from build123d import *

# Parameters (mm, degrees)
SKETCH1_W           = 50
SKETCH1_H           = 50
BOSS_EXTRUDE1_DEPTH = 1439.7
SKETCH2_W           = 50
SKETCH2_H           = 60
BOSS_EXTRUDE2_DEPTH = 100
SKETCH3_W           = 250
SKETCH3_H           = 60
SKETCH3_W_2         = 50
BOSS_EXTRUDE3_DEPTH = 15
SKETCH4_R           = 10
CUT_EXTRUDE1_DEPTH  = 1474.001542864
SKETCH5_R           = 15
CUT_EXTRUDE2_DEPTH  = 1477.156207783
SKETCH7_R           = 15
CUT_EXTRUDE3_DEPTH  = 1477.156207783


with BuildPart() as part:
    # Sketch1 → Boss-Extrude1 (new body)
    with BuildSketch(Plane(origin=(0, 0, 0), x_dir=(1, 0, 0), z_dir=(0, 1, 0))):
        with Locations((-56.349206349, -14.484126984)):
            Rectangle(SKETCH1_W, SKETCH1_H)
    extrude(amount=BOSS_EXTRUDE1_DEPTH)

    # Sketch2 → Boss-Extrude2 (add)
    with BuildSketch(Plane(origin=(-31.349206349, 0, 0), x_dir=(0, 0, -1), z_dir=(1, 0, 0))):
        with Locations((-14.484126984, 1409.7)):
            Rectangle(SKETCH2_W, SKETCH2_H)
        with Locations((-14.484126984, 30)):
            Rectangle(SKETCH2_W, SKETCH2_H)
    extrude(amount=BOSS_EXTRUDE2_DEPTH)

    # Sketch3 → Boss-Extrude3 (add)
    with BuildSketch(Plane(origin=(68.650793651, 0, 0), x_dir=(0, 0, -1), z_dir=(1, 0, 0))):
        with Locations((-164.484126984, 30)):
            Rectangle(SKETCH3_W, SKETCH3_H)
        with Locations((135.515873016, 30)):
            Rectangle(SKETCH3_W, SKETCH3_H)
        with Locations((-164.484126984, 1409.7)):
            Rectangle(SKETCH3_W, SKETCH3_H)
        with Locations((135.515873016, 1409.7)):
            Rectangle(SKETCH3_W, SKETCH3_H)
        with Locations((-14.484126984, 1409.7)):
            Rectangle(SKETCH3_W_2, SKETCH3_H)
        with Locations((-14.484126984, 30)):
            Rectangle(SKETCH3_W_2, SKETCH3_H)
    extrude(amount=BOSS_EXTRUDE3_DEPTH)

    # Sketch4 → Cut-Extrude1 (cut, through all)
    with BuildSketch(Plane.XY.offset(39.484126984)):
        with Locations((-56.577927761, 597.467393714)):
            Circle(SKETCH4_R)
        with Locations((-56.577927761, 527.467393714)):
            Circle(SKETCH4_R)
        with Locations((-56.577927761, 457.467393714)):
            Circle(SKETCH4_R)
        with Locations((-56.577927761, 387.467393714)):
            Circle(SKETCH4_R)
        with Locations((-56.577927761, 317.467393714)):
            Circle(SKETCH4_R)
        with Locations((-56.577927761, 247.467393714)):
            Circle(SKETCH4_R)
        with Locations((-56.577927761, 177.467393714)):
            Circle(SKETCH4_R)
        with Locations((-56.577927761, 107.467393714)):
            Circle(SKETCH4_R)
        with Locations((-56.577927761, 667.467393714)):
            Circle(SKETCH4_R)
        with Locations((-56.577927761, 737.467393714)):
            Circle(SKETCH4_R)
    extrude(amount=-CUT_EXTRUDE1_DEPTH, mode=Mode.SUBTRACT)

    # Sketch5 → Cut-Extrude2 (cut, through all)
    with BuildSketch(Plane.ZY.offset(-68.650793651)):
        with Locations((-228.539538752, 1409.7)):
            Circle(SKETCH5_R)
        with Locations((-168.539538752, 1409.7)):
            Circle(SKETCH5_R)
        with Locations((-108.539538752, 1409.7)):
            Circle(SKETCH5_R)
        with Locations((-48.539538752, 1409.7)):
            Circle(SKETCH5_R)
        with Locations((247.647169752, 1409.7)):
            Circle(SKETCH5_R)
        with Locations((187.647169752, 1409.7)):
            Circle(SKETCH5_R)
        with Locations((127.647169752, 1409.7)):
            Circle(SKETCH5_R)
        with Locations((67.647169752, 1409.7)):
            Circle(SKETCH5_R)
    extrude(amount=-CUT_EXTRUDE2_DEPTH, mode=Mode.SUBTRACT)

    # Sketch7 → Cut-Extrude3 (cut, through all)
    with BuildSketch(Plane.ZY.offset(-68.650793651)):
        with Locations((-230.917241816, 30)):
            Circle(SKETCH7_R)
        with Locations((-170.917241816, 30)):
            Circle(SKETCH7_R)
        with Locations((-110.917241816, 30)):
            Circle(SKETCH7_R)
        with Locations((-50.917241816, 30)):
            Circle(SKETCH7_R)
        with Locations(Location((78.601472043, 30, 0), (0, 0, 180))):
            Circle(SKETCH7_R)
        with Locations(Location((138.601472043, 30, 0), (0, 0, 180))):
            Circle(SKETCH7_R)
        with Locations(Location((198.601472043, 30, 0), (0, 0, 180))):
            Circle(SKETCH7_R)
        with BuildLine():
            ThreePointArc((259.111313866, 44.991332873), (244.62115569, 30), (259.111313866, 15.008667127))
            ThreePointArc((259.111313866, 15.008667127), (273.601472043, 30), (259.111313866, 44.991332873))
        make_face()
    extrude(amount=-CUT_EXTRUDE3_DEPTH, mode=Mode.SUBTRACT)


solid = part.part
The model under review builds one solid part; all positions refer to its coordinate system, in mm. A direction names the side the tool comes from. Round coordinates to 2 decimals unless told otherwise and drop trailing zeros. Write each loop counter-clockwise with the first axis right and the second up, starting at its lowest first coordinate (ties: lowest second). Pieces come first, ordered by that corner, then holes. Notation, with made-up numbers: M 22.25,52 L 49.25,52 A13 cw 49.25,61 Z; hole C 60,-13.75 d10. An arc over 180 degrees is marked long. Answer as CSV lines item,"result". Start each with the question number.
Q1. Wall thickness on line 1 along Y through (x, z) = (26.5, -2); line 2 along Z through (x, y) = (-67, 657.5); line 3 along X through (y, z) = (94, -3): over which ranges is each line inside the solid? List them lowest first.
Q2. Tool access review of faces 1 (the face through (-40, 716, 39.484)), 2 (the face through (51, 1379.7, 16)), 3 (the face through (68.651, 1410, -134)): name each direction out of +Z, -Z, +X, -X, +Y, -Y from which nothing blocks a thin tool from reaching the whole face with its end or side.
Q3. Consider section A-A, the plane x = -9.5. Give the boundary of the cut face in (y, z), then the cut area to 3 significant figures.
Q4. Clearance check with flat-ended pins moving along their axes: P1, Ø12, axis at x = -56.58, y = 597.47, coming from the -Z side; P2, Ø10, axis at x = -34.5, y = 1265.5, coming from the -Z side. State where each tip first meets the part, or that it passes through.
Q5. Consider section B-B, the plane y = 30. State how many separate pieces and enclosed holes the cut face has, then the cut area to 3 significant figures.
Q6. Consider section C-C, the plane y = 931. Give the boundary of the cut face in (x, z), then the cut area to 3 significant figures.
Q7. The part is to be moulded in two halves that separate along Y. For faces 4 (the face through (25, 1439.7, 16)), 5 (the face through (76.05, 1410.36, 112.66)), 6 (the face through (68.651, 30, -134)), say which applies: +Y half, -Y half, draft (parallel to the pull), parting line (faces both ways), or undercut.
Result set:
1,line 1,"y = 0 to 60, 1379.7 to 1439.7"
1,line 2,"z = -10.52 to 39.48"
1,line 3,"x = -81.35 to -31.35"
2,face 1,"+Z, -X, +Y, -Y"
2,face 2,"+Z, -Z, +X"
2,face 3,"-Z, -X, +Y, -Y"
3,outline,"M 0,-10.52 L 60,-10.52 L 60,39.48 L 0,39.48 Z; M 1379.7,-10.52 L 1439.7,-10.52 L 1439.7,39.48 L 1379.7,39.48 Z"
3,area,"6,000 mm²"
4,P1,"passes through"
4,P2,"stops at z = -10.52"
5,separate pieces,"9"
5,enclosed holes,"0"
5,area,"12,200 mm²"
6,outline,"M -81.35,-10.52 L -31.35,-10.52 L -31.35,39.48 L -81.35,39.48 Z"
6,area,"2,500 mm²"
7,face 4,"+Y half"
7,face 5,"undercut"
7,face 6,"draft"
